Verification items for the finished model (mm, model axes). Face numbers are marked on the shaded views. A direction names the side the tool comes from. Round coordinates to 2 decimals unless told otherwise and drop trailing zeros. Write each loop counter-clockwise with the first axis right and the second up, starting at its lowest first coordinate (ties: lowest second). Pieces come first, ordered by that corner, then holes. Notation, with made-up numbers: (83, -3.5) -> (112, -3.5) arc R14 ccw to (112, 2.5) -> close; hole circle Ø1 at (-12.75, 86). An arc over 180 degrees is marked (long way). Answer as a JSON object with one key per item and string values. Group by question number.
(1) Set-up check for the marked faces 1, 2 and 3: record each of +Z, -Z, +X, -X, +Y, -Y from which the full face is reachable in a straight line by a thin tool's end or side.
(2) Sectioned sample at C-C on z = 0.75. Record the cut outline in (x, y).
(3) Scan lines: L1, parallel to X at y = 1.95, z = -2; L2, parallel to Z at x = -10.25, y = 0.65; L3, parallel to Z at x = -11.25, y = 2.5. Record each from-to range of solid material in increasing order. Write a range as from..to.
(4) Sectioned sample at B-B on y = 1.9. Record the cut outline in (x, z), and give its area (3 significant figures).
(5) Sectioned sample at D-D on x = -17.5. Record the cut outline in (y, z), and give its area (3 significant figures).
(6) Draft check along Z on the marked faces 4, 5 and 6. Enter one of: released by +Z, released by -Z, zero draft, split by the parting line, or undercut.
(7) Gauge pin test, flat end, axial feed: pin 1 Ø4 at (x, z) = (-9.5, -1) entering from +Y. Record the tip position at first contact, or that the pin passes through.
(8) Sectioned sample at A-A on z = -2. Record the cut outline in (x, y), and give its area (3 significant figures).
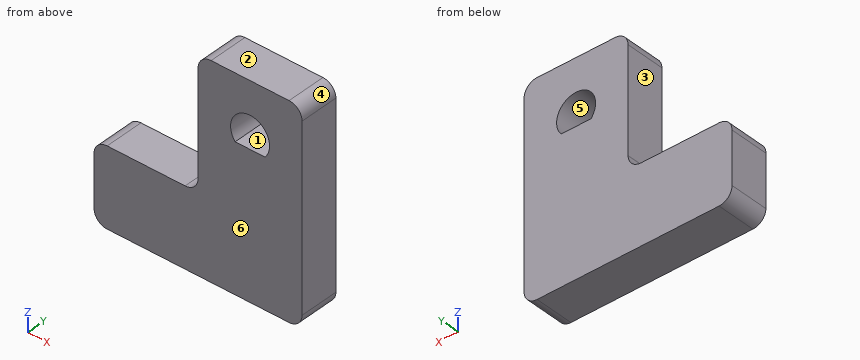
```python
from build123d import *

# Parameters (mm, degrees)
BOSS_EXTRUDE2_DEPTH = 3
FILLET1_R           = 1
FILLET2_R           = 1
FILLET3_R           = 1
FILLET4_R           = 1
FILLET5_R           = 1
FILLET6_R           = 1
CUT_EXTRUDE2_DEPTH  = 3


with BuildPart() as part:
    # Sketch1 → Boss-Extrude2 (new body)
    with BuildSketch(Plane(origin=(0, 0, 0), x_dir=(1, 0, 0), z_dir=(0, 1, 0))):
        Polygon((-6.234693371, -2), (-14.234693371, -2), (-14.234693371, 8), (-22.234693371, 8), (-22.234693371, 14), (-6.234693371, 14), (-6.234693371, 8), align=None)
    extrude(amount=BOSS_EXTRUDE2_DEPTH)

    # Fillet1
    fillet1_edges = [part.edges().sort_by_distance(p)[0] for p in [
        (-22.234693371, 1.5, -14),
    ]]
    fillet(fillet1_edges, radius=FILLET1_R)

    # Fillet2
    fillet2_edges = [part.edges().sort_by_distance(p)[0] for p in [
        (-22.234693371, 1.5, -8),
    ]]
    fillet(fillet2_edges, radius=FILLET2_R)

    # Fillet3
    fillet3_edges = [part.edges().sort_by_distance(p)[0] for p in [
        (-6.234693371, 1.5, -14),
    ]]
    fillet(fillet3_edges, radius=FILLET3_R)

    # Fillet4
    fillet4_edges = [part.edges().sort_by_distance(p)[0] for p in [
        (-14.234693371, 1.5, 2),
    ]]
    fillet(fillet4_edges, radius=FILLET4_R)

    # Fillet5
    fillet5_edges = [part.edges().sort_by_distance(p)[0] for p in [
        (-6.234693371, 1.5, 2),
    ]]
    fillet(fillet5_edges, radius=FILLET5_R)

    # Fillet6
    fillet6_edges = [part.edges().sort_by_distance(p)[0] for p in [
        (-14.234693371, 1.5, -8),
    ]]
    fillet(fillet6_edges, radius=FILLET6_R)

    # Sketch3 → Cut-Extrude2 (cut)
    with BuildSketch(Plane(origin=(0, 3, 0), x_dir=(1, 0, 0), z_dir=(0, 1, 0))):
        with BuildLine():
            Line((-11.383221505, 2.964822846), (-9.086165237, 2.964822846))
            ThreePointArc((-9.086165237, 2.964822846), (-10.234693371, 0.5), (-11.383221505, 2.964822846))
        make_face()
    extrude(amount=-CUT_EXTRUDE2_DEPTH, mode=Mode.SUBTRACT)


solid = part.part
```
Computed values:
{
 "1": {"face 1": "+Y, -Y", "face 2": "+Z, +X, -X, +Y, -Y", "face 3": "+Z, -X, +Y, -Y"},
 "2": {"outline": "(-14.23, 0) -> (-6.23, 0) -> (-6.23, 3) -> (-14.23, 3) -> close"},
 "3": {"L1": "-14.23..-11.73, -8.73..-6.23", "L2": "-14..-2.96, -0.5..2", "L3": "-14..-2.96, -0.9..2"},
 "4": {"outline": "(-22.23, -13) arc R1 ccw to (-21.23, -14) -> (-7.23, -14) arc R1 ccw to (-6.23, -13) -> (-6.23, 1) arc R1 ccw to (-7.23, 2) -> (-13.23, 2) arc R1 ccw to (-14.23, 1) -> (-14.23, -7) arc R1 cw to (-15.23, -8) -> (-21.23, -8) arc R1 ccw to (-22.23, -9) -> close; hole (-11.38, -2.96) -> (-9.09, -2.96) arc R1.5 ccw (long way) to start", "area": "169 mm2"},
 "5": {"outline": "(0, -14) -> (3, -14) -> (3, -8) -> (0, -8) -> close", "area": "18.0 mm2"},
 "6": {"face 4": "released by +Z", "face 5": "undercut", "face 6": "zero draft"},
 "7": {"pin 1": "y = 3"},
 "8": {"outline": "(-14.23, 0) -> (-11.73, 0) -> (-11.73, 3) -> (-14.23, 3) -> close; (-8.73, 0) -> (-6.23, 0) -> (-6.23, 3) -> (-8.73, 3) -> close", "area": "15.0 mm2"}
}
